```python
from build123d import *

# Parameters (mm, degrees)
SKETCH_1_W          = 7.85
SKETCH_1_H          = 7.85
EXTRUDE_1_DEPTH     = 10
SKETCH_2_W          = 10
SKETCH_2_H          = 10
EXTRUDE_2_DEPTH     = 30
CUT_EXTRUDE_1_DEPTH = 30
FILLET_1_R          = 1
CHAMFER_1_SIZE      = 1
SKETCH_4_R          = 1.45
CUT_EXTRUDE_2_DEPTH = 30


with BuildPart() as part:
    # ｽｹｯﾁ1 → ﾎﾞｽ - 押し出し1 (new body)
    with BuildSketch(Plane(origin=(0, 0, 0), x_dir=(1, 0, 0), z_dir=(0, 1, 0))):
        Rectangle(SKETCH_1_W, SKETCH_1_H)
    extrude(amount=EXTRUDE_1_DEPTH)

    # ｽｹｯﾁ2 → ﾎﾞｽ - 押し出し2 (add)
    with BuildSketch(Plane(origin=(0, 10, 0), x_dir=(1, 0, 0), z_dir=(0, 1, 0))):
        Rectangle(SKETCH_2_W, SKETCH_2_H)
    extrude(amount=EXTRUDE_2_DEPTH)

    # ｽｹｯﾁ3 → ｶｯﾄ - 押し出し1 (cut)
    with BuildSketch(Plane.XY.offset(5)):
        Polygon((-5, 27.320508076), (5, 10), (5, 40), (-5, 40), align=None)
    extrude(amount=-CUT_EXTRUDE_1_DEPTH, mode=Mode.SUBTRACT)

    # ﾌｨﾚｯﾄ1
    fillet_1_edges = [part.edges().sort_by_distance(p)[0] for p in [
        (-5, 27.320508076, 0),
    ]]
    fillet(fillet_1_edges, radius=FILLET_1_R)

    # 面取り1
    chamfer_1_edges = [part.edges().sort_by_distance(p)[0] for p in [
        (0, 0, 3.925),
        (-3.925, 0, 0),
        (0, 0, -3.925),
        (3.925, 0, 0),
    ]]
    chamfer(chamfer_1_edges, length=CHAMFER_1_SIZE)

    # ｽｹｯﾁ4 → ｶｯﾄ - 押し出し2 (cut)
    with BuildSketch(Plane.XY.offset(3.925)):
        with Locations((0, 5)):
            Circle(SKETCH_4_R)
    extrude(amount=-CUT_EXTRUDE_2_DEPTH, mode=Mode.SUBTRACT)


solid = part.part
```
Geometry check sheet. Reference: the model listing, model coordinates, mm. A direction names the side the tool comes from. Give positions to 0.01 mm unless a question says otherwise; leave off trailing zeros. Write each loop counter-clockwise with the first axis right and the second up, starting at its lowest first coordinate (ties: lowest second). Pieces come first, ordered by that corner, then holes.
1) Material ranges on L1, parallel to Z at x = 1, y = 8 (3 decimals); L2, parallel to Y at x = 0, z = -1; L3, parallel to X at y = 12.5, z = 0.5, recorded low to high.
2) Access from +Z, -Z, +X, -X, +Y, -Y to the whole of each face (thin tool, end or side, straight path). Record for faces 1 (the flat face through (3.925, 5, 0)), 2 (the flat face through (0.8, 6.4, 3.925)), 3 (the flat face through (-3.925, 5, 0)).
3) Section check C-C, the plane z = -1.75. Record the boundary of the cut face in (x, y) (3 decimals).
4) Section check B-B, the plane x = -0.75. Record the boundary of the cut face in (y, z) (3 decimals).
5) Section check D-D, the plane y = 7.75. Record the boundary of the cut face in (x, z) (3 decimals), and give its area (3 significant figures).
6) Release check for a two-part mould opening along X. For faces 4 (the flat face through (0.9, 17.1, 0.1)), 5 (the flat face through (-1, 16, -5)), 6 (the cylindrical face through (-0.314, 3.584, 0.055)), 7 (the flat face through (-3.418, 0.493, 0.055)) record: pulls with the +X half, pulls with the -X half, needs draft (parallel to the pull), parting line crosses it, or undercut.
7) Section check A-A, the plane y = 5. Record the boundary of the cut face in (x, z) (3 decimals), and give its area (3 significant figures).
8) Gauge pin test, flat ends, axial feed: pin 1 (2 mm diameter, centred on y = 3.5, z = 4, fed in from +X) (3 decimals); pin 2 (4 mm diameter, centred on y = 6.5, z = -1.5, fed in from -X) (3 decimals); pin 3 (5 mm diameter, centred on x = 2.5, z = -1, fed in from +Y). Record the tip position at first contact, or that the pin passes through.
Computed:
1. L1: z = -3.925 to 3.925
1. L2: y = 0 to 3.55, 6.45 to 18.66
1. L3: x = -5 to 3.56
2. face 1: +Z, -Z, +X, -Y
2. face 2: +Z, +X, -X, -Y
2. face 3: +Z, -Z, -X, -Y
3. outline: (-5, 10) - (-3.925, 10) - (-3.925, 1) - (-2.925, 0) - (2.925, 0) - (3.925, 1) - (3.925, 10) - (5, 10) - (-3.134, 24.088) arc R1 ccw to (-5, 23.588) - close; hole circle Ø2.9 at (0, 5)
4. outline: (0, -2.925) - (1, -3.925) - (3.759, -3.925) - (3.759, 3.925) - (1, 3.925) - (0, 2.925) - close; (6.241, -3.925) - (10, -3.925) - (10, -5) - (19.959, -5) - (19.959, 5) - (10, 5) - (10, 3.925) - (6.241, 3.925) - close
5. outline: (-3.925, -3.925) - (3.925, -3.925) - (3.925, 3.925) - (-3.925, 3.925) - close
5. area: 61.6 mm2
6. face 4: pulls with the +X half
6. face 5: needs draft
6. face 6: undercut
6. face 7: pulls with the -X half
7. outline: (-3.925, -3.925) - (-1.45, -3.925) - (-1.45, 3.925) - (-3.925, 3.925) - close; (1.45, -3.925) - (3.925, -3.925) - (3.925, 3.925) - (1.45, 3.925) - close
7. area: 38.9 mm2
8. pin 1: stops at x = 3.925
8. pin 2: stops at x = -3.925
8. pin 3: stops at y = 18.66
